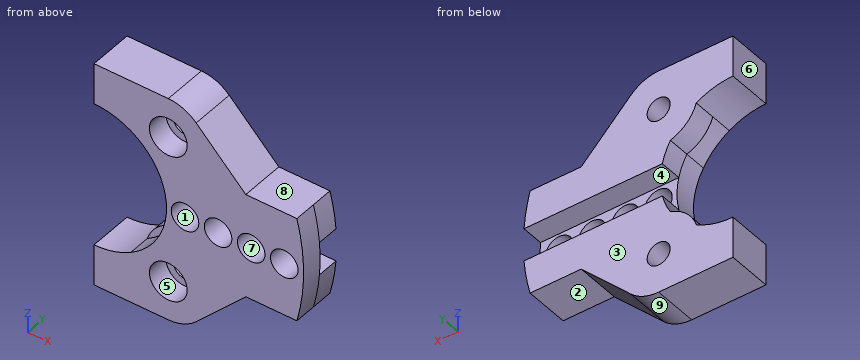
from build123d import *
from build123d.topology import SkipClean

# Parameters (mm, degrees)
SKETCH1_R           = 2.0828
SKETCH1_R_2         = 2.5
BOSS_EXTRUDE2_DEPTH = 4
BOSS_EXTRUDE3_START = 4
SKETCH5_R           = 3.429
SKETCH5_R_2         = 2.5
BOSS_EXTRUDE3_DEPTH = 4
CUT_EXTRUDE2_START  = -4
CUT_EXTRUDE2_DEPTH  = 4


with BuildPart() as part:
    # Sketch1 → Boss-Extrude2 (new body)
    with BuildSketch(Plane(origin=(0, 0, 0), x_dir=(1, 0, 0), z_dir=(0, 1, 0))):
        with BuildLine():
            Line((0, 20.614134159), (0, 13.151202806))
            ThreePointArc((0, 13.151202806), (3.445207277, 12.691914043), (6.64977573, 11.346127885))
            ThreePointArc((6.64977573, 11.346127885), (8.418990091, 8.418990091), (11.346127885, 6.64977573))
            ThreePointArc((11.346127885, 6.64977573), (13.151202806, 0), (11.346127885, -6.64977573))
            ThreePointArc((11.346127885, -6.64977573), (8.418990091, -8.418990091), (6.64977573, -11.346127885))
            ThreePointArc((6.64977573, -11.346127885), (3.445207277, -12.691914043), (0, -13.151202806))
            Line((0, -13.151202806), (0, -20.614134159))
            Line((0, -20.614134159), (13.470384159, -20.614134159))
            ThreePointArc((13.470384159, -20.614134159), (16.204178929, -20.070348569), (18.521778227, -18.521778227))
            Line((18.521778227, -18.521778227), (27.518556454, -9.525))
            Line((27.518556454, -9.525), (36.786877756, -9.525))
            ThreePointArc((36.786877756, -9.525), (38, 0), (36.786877756, 9.525))
            Line((36.786877756, 9.525), (27.518556454, 9.525))
            Line((27.518556454, 9.525), (18.521778227, 18.521778227))
            ThreePointArc((18.521778227, 18.521778227), (16.204178929, 20.070348569), (13.470384159, 20.614134159))
            Line((13.470384159, 20.614134159), (0, 20.614134159))
        make_face()
        with Locations(Location((13.470384159, 13.470384159, 0), (0, 0, 270))):
            Circle(SKETCH1_R, mode=Mode.SUBTRACT)
        with Locations(Location((13.470384159, -13.470384159, 0), (0, 0, 90))):
            Circle(SKETCH1_R, mode=Mode.SUBTRACT)
        with Locations(Location((16.5, 0, 0), (0, 0, 270))):
            Circle(SKETCH1_R_2, mode=Mode.SUBTRACT)
        with Locations(Location((22.5, 0, 0), (0, 0, 270))):
            Circle(SKETCH1_R_2, mode=Mode.SUBTRACT)
        with Locations(Location((28.5, 0, 0), (0, 0, 270))):
            Circle(SKETCH1_R_2, mode=Mode.SUBTRACT)
        with Locations(Location((34.5, 0, 0), (0, 0, 270))):
            Circle(SKETCH1_R_2, mode=Mode.SUBTRACT)
    extrude(amount=BOSS_EXTRUDE2_DEPTH)

    # Sketch5 → Boss-Extrude3 (add)
    with SkipClean():  # the faces are left unmerged after this step: merging them gives an invalid solid
        with BuildSketch(Plane.XZ.offset(BOSS_EXTRUDE3_START)):
            with BuildLine():
                ThreePointArc((36.786877756, -9.525), (38, 0), (36.786877756, 9.525))
                Line((36.786877756, 9.525), (27.518556454, 9.525))
                Line((27.518556454, 9.525), (18.521778227, 18.521778227))
                ThreePointArc((18.521778227, 18.521778227), (16.204178929, 20.070348569), (13.470384159, 20.614134159))
                Line((13.470384159, 20.614134159), (0, 20.614134159))
                Line((0, 20.614134159), (0, 13.151202806))
                ThreePointArc((0, 13.151202806), (3.445207277, 12.691914043), (6.64977573, 11.346127885))
                ThreePointArc((6.64977573, 11.346127885), (9.299304685, 9.299304685), (11.346127885, 6.64977573))
                ThreePointArc((11.346127885, 6.64977573), (13.151202806, 0), (11.346127885, -6.64977573))
                ThreePointArc((11.346127885, -6.64977573), (9.299304685, -9.299304685), (6.64977573, -11.346127885))
                ThreePointArc((6.64977573, -11.346127885), (3.445207277, -12.691914043), (0, -13.151202806))
                Line((0, -13.151202806), (0, -20.614134159))
                Line((0, -20.614134159), (13.470384159, -20.614134159))
                ThreePointArc((13.470384159, -20.614134159), (16.204178929, -20.070348569), (18.521778227, -18.521778227))
                Line((18.521778227, -18.521778227), (27.518556454, -9.525))
                Line((27.518556454, -9.525), (36.786877756, -9.525))
            make_face()
            with Locations(Location((13.470384159, -13.470384159, 0), (0, 0, 270))):
                Circle(SKETCH5_R, mode=Mode.SUBTRACT)
            with Locations(Location((16.5, 0, 0), (0, 0, 270))):
                Circle(SKETCH5_R_2, mode=Mode.SUBTRACT)
            with Locations(Location((13.470384159, 13.470384159, 0), (0, 0, 270))):
                Circle(SKETCH5_R, mode=Mode.SUBTRACT)
            with BuildLine():
                ThreePointArc((25, 0), (22.5, -2.5), (20, 0))
                ThreePointArc((20, 0), (22.5, 2.5), (25, 0))
            make_face(mode=Mode.SUBTRACT)
            with BuildLine():
                ThreePointArc((31, 0), (28.5, -2.5), (26, 0))
                ThreePointArc((26, 0), (28.5, 2.5), (31, 0))
            make_face(mode=Mode.SUBTRACT)
            with BuildLine():
                ThreePointArc((37, 0), (34.5, -2.5), (32, 0))
                ThreePointArc((32, 0), (34.5, 2.5), (37, 0))
            make_face(mode=Mode.SUBTRACT)
        extrude(amount=-BOSS_EXTRUDE3_DEPTH)

    # Sketch6 → Cut-Extrude2 (cut)
    with SkipClean():  # the faces are left unmerged after this step: merging them gives an invalid solid
        with BuildSketch(Plane(origin=(0, 4, 0), x_dir=(1, 0, 0), z_dir=(0, 1, 0)).offset(CUT_EXTRUDE2_START)):
            with BuildLine():
                Line((12.804457632, -3), (37.88139385, -3))
                ThreePointArc((37.88139385, -3), (38, 0), (37.88139385, 3))
                Line((37.88139385, 3), (12.804457632, 3))
                ThreePointArc((12.804457632, 3), (13.151202806, 0), (12.804457632, -3))
            make_face()
        extrude(amount=CUT_EXTRUDE2_DEPTH, mode=Mode.SUBTRACT)


solid = part.part
Design review of the part built by this model. Coordinates are the model's own, in mm. Face numbers are marked on the shaded views. A direction names the side the tool comes from. Round coordinates to 2 decimals unless told otherwise and drop trailing zeros. Loops run counter-clockwise (first coordinate to the right, second up) from the corner with the lowest first, then second, coordinate; pieces in that order, holes last. Notation, with made-up numbers: (-28, 58.5) - (24, 58.5) arc R6 ccw to (24, 64.5) - close; hole circle Ø2 at (60.5, 18). An arc over 180 degrees is marked (long way). One line per item, written item: value. Start each with the question number.
1) To check wall thickness, follow L1, parallel to Z at x = 34.5, y = 1.5 (3 decimals); L2, parallel to Z at x = 23, y = -0.25; L3, parallel to X at y = -1.75, z = -16.5. State the ranges of each line that lie inside material, in increasing order. Write a range as from..to.
2) Consider section A-A on y = 1.5. Give the boundary of the cut face in (x, z) (1 decimal), then the cut area to 3 significant figures.
3) Draft analysis for pull direction Z (two halves, no side actions). For the marked faces 6, 7, 8 and 9, state which applies: +Z half, -Z half, draft (parallel to the pull), parting line (faces both ways), or undercut.
4) Insertion check: pin 1 Ø1.5 at (y, z) = (2, 11) entering from +X; pin 2 Ø11 at (x, z) = (13.47, 13.47) entering from -Y; pin 3 Ø4 at (y, z) = (-0.5, 1) entering from -X; pin 4 Ø3 at (x, y) = (20, 1) entering from +Z. Each pin has a flat end and moves straight along its axis. Give the tip position at first contact, or say it passes through.
5) Consider section D-D on y = -1.75. Give the boundary of the cut face in (x, z) (1 decimal), then the cut area to 3 significant figures.
6) For the marked faces 1, 2, 3, 4 and 5, list the 3-axis set-ups (+Z, -Z, +X, -X, +Y, -Y) from which the entire face can be reached by the end or side of a thin tool; tool diameter is ignored.
7) Consider section B-B on x = 28.5. Give the boundary of the cut face in (y, z) (3 decimals).
8) Consider section C-C on z = 0. Give the boundary of the cut face in (x, y), then the cut area to 3 significant figures.
Reported:
1. L1: z = -9.525..-3, 3..9.525
1. L2: z = -14.04..-2.45, 2.45..14.04
1. L3: x = 0..11.86, 15.08..20.54
2. outline: (0, -20.6) - (13.5, -20.6) arc R7.1 ccw to (18.5, -18.5) - (27.5, -9.5) - (36.8, -9.5) arc R38 ccw to (37.9, -3) - (12.8, -3) arc R13.2 cw to (11.3, -6.6) arc R7.1 ccw to (6.6, -11.3) arc R13.2 cw to (0, -13.2) - close; (0, 13.2) arc R13.2 cw to (6.6, 11.3) arc R7.1 ccw to (11.3, 6.6) arc R13.2 cw to (12.8, 3) - (37.9, 3) arc R38 ccw to (36.8, 9.5) - (27.5, 9.5) - (18.5, 18.5) arc R7.1 ccw to (13.5, 20.6) - (0, 20.6) - close; hole circle Ø4.2 at (13.5, -13.5); hole circle Ø4.2 at (13.5, 13.5)
2. area: 764 mm^2
3. face 6: draft
3. face 7: undercut
3. face 8: +Z half
3. face 9: -Z half
4. pin 1: stops at x = 26.79
4. pin 2: stops at y = -4
4. pin 3: stops at x = 12.8
4. pin 4: stops at z = 18.54
5. outline: (0, -20.6) - (13.5, -20.6) arc R7.1 ccw to (18.5, -18.5) - (27.5, -9.5) - (36.8, -9.5) arc R38 ccw to (36.8, 9.5) - (27.5, 9.5) - (18.5, 18.5) arc R7.1 ccw to (13.5, 20.6) - (0, 20.6) - (0, 13.2) arc R13.2 cw to (0, -13.2) - close; hole circle Ø6.9 at (13.5, -13.5); hole circle Ø6.9 at (13.5, 13.5); hole circle Ø5 at (16.5, 0); hole circle Ø5 at (22.5, 0); hole circle Ø5 at (28.5, 0); hole circle Ø5 at (34.5, 0)
5. area: 777 mm^2
6. face 1: +Y, -Y
6. face 2: -Z, +X, +Y, -Y
6. face 3: +Z, -Z, +X, -X, +Y
6. face 4: +X, -X, +Y
6. face 5: -Y
7. outline: (-4, -9.525) - (4, -9.525) - (4, -3) - (0, -3) - (0, -2.5) - (-4, -2.5) - close; (-4, 2.5) - (0, 2.5) - (0, 3) - (4, 3) - (4, 9.525) - (-4, 9.525) - close
8. outline: (13.15, -4) - (14, -4) - (14, 0) - (13.15, 0) - close; (19, -4) - (20, -4) - (20, 0) - (19, 0) - close; (25, -4) - (26, -4) - (26, 0) - (25, 0) - close; (31, -4) - (32, -4) - (32, 0) - (31, 0) - close; (37, -4) - (38, -4) - (38, 0) - (37, 0) - close
8. area: 19.4 mm^2
